from build123d import *

# Parameters (mm, degrees)
F1_DEPTH       = 4
F3_D           = 3.1
F3_CBORE_D     = 6.2
F3_CBORE_DEPTH = 1
F4_W           = 1.5
F4_H           = 7
F5_DEPTH       = 10
F6_SIZE        = 1.5
F7_R           = 2


with BuildPart() as f1:
    # F0 (on Front) → F1 (new body)
    with BuildSketch(Plane.XZ):
        Polygon((-17, 0), (8, 0), (8, 30), (0, 30), (0, 7), (-17, 7), align=None)
    extrude(amount=F1_DEPTH)

    # F3 (through all)
    with Locations(Plane.XZ.offset(4)):
        with Locations((4, 25), (4, 5)):
            CounterBoreHole(F3_D / 2, F3_CBORE_D / 2, F3_CBORE_DEPTH)

    # F4 (on Front) → F5 (join)
    with BuildSketch(Plane.XZ):
        with Locations((-16.25, 3.5)):
            Rectangle(F4_W, F4_H)
    extrude(amount=-F5_DEPTH)

    # F6
    f6_edges = [f1.edges().sort_by_distance(p)[0] for p in [
        (8, 0, 15),
    ]]
    chamfer(f6_edges, length=F6_SIZE)

    # F7
    f7_edges = [f1.edges().sort_by_distance(p)[0] for p in [
        (-15.5, 0, 3.5),
        (0, -2, 7),
    ]]
    fillet(f7_edges, radius=F7_R)


solid = f1.part
Model file for the job. Use its own axes, mm. A direction names the side the tool comes from. Give positions to 0.01 mm unless a question says otherwise; leave off trailing zeros. Loops run counter-clockwise (first coordinate to the right, second up) from the corner with the lowest first, then second, coordinate; pieces in that order, holes last.
Item 1: Drill centre lines: line 1 along Z through (x, y) = (4, -3.2); line 2 along Z through (x, y) = (4, -1.85); line 3 along X through (y, z) = (-1.5, 15). Where is each one in solid material? Low to high.
Check values:
line 1: z = 0 to 1.9, 8.1 to 21.9, 28.1 to 30
line 2: z = 0 to 3.45, 6.55 to 23.45, 26.55 to 30
line 3: x = 0 to 8
Item 2: Slice it at B-B (y = -2.25). Write the cut outline in (x, z).
Check values:
outline: (-17, 0) - (8, 0) - (8, 30) - (0, 30) - (0, 9) arc R2 cw to (-2, 7) - (-17, 7) - close; hole circle Ø3.1 at (4, 5); hole circle Ø3.1 at (4, 25)
Item 3: Slice it at C-C (x = 4). Write the cut outline in (y, z).
Check values:
outline: (-4, 0) - (0, 0) - (0, 3.45) - (-3, 3.45) - (-3, 1.9) - (-4, 1.9) - close; (-4, 8.1) - (-3, 8.1) - (-3, 6.55) - (0, 6.55) - (0, 23.45) - (-3, 23.45) - (-3, 21.9) - (-4, 21.9) - close; (-4, 28.1) - (-3, 28.1) - (-3, 26.55) - (0, 26.55) - (0, 30) - (-4, 30) - close
Item 4: Drop flat-ended pins along their axis: P1, Ø3, axis at x = 4, z = 25, coming from the +Y side; P2, Ø1.9, axis at x = 3, z = 3.5, coming from the -Y side; P3, Ø7, axis at x = 4, z = 5, coming from the +Y side; P4, Ø6, axis at x = -3, y = 2, coming from the +Z side. Give the stop position or say it passes through.
Check values:
P1: passes through
P2: stops at y = -3
P3: stops at y = 0
P4: stops at z = 7.43
Item 5: Slice it at D-D (z = 11.5). Write the cut outline in (x, y).
Check values:
outline: (0, -4) - (8, -4) - (8, -1.5) - (6.5, 0) - (0, 0) - close
Item 6: Which spindle directions (+Z, -Z, +X, -X, +Y, -Y) get a long thin tool onto all of the face, cutting with end or side? Do faces 1 (the face through (0, -2, 20)), 2 (the face through (3.328, -3.507, 1.974)), 3 (the face through (-15.5, 6, 3)). Say none if no direction does.
Check values:
face 1: +Z, -X, +Y, -Y
face 2: -Y
face 3: +Z, -Z, +X, +Y
Item 7: Mould opens along Z. For faces 4 (the face through (-11.3, -0.2, 7)), 5 (the face through (5.55, -1.48, 5.07)), 6 (the face through (7.3, -0.8, 14.8)), 7 (the face through (-7.5, -0.2, 0)) say: +Z half, -Z half, draft (parallel to the pull), parting line (faces both ways), or undercut.
Check values:
face 4: +Z half
face 5: undercut
face 6: draft
face 7: -Z half
Item 8: Slice it at A-A (z = 25). Write the cut outline in (x, y).
Check values:
outline: (0, -4) - (0.9, -4) - (0.9, -3) - (2.45, -3) - (2.45, 0) - (0, 0) - close; (5.55, -3) - (7.1, -3) - (7.1, -4) - (8, -4) - (8, -1.5) - (6.5, 0) - (5.55, 0) - close
